CAD build for the part. Positions are in the model's coordinates, mm. Face numbers are marked on the shaded views. A direction names the side the tool comes from. Coordinates: 2 decimals unless noted, no trailing zeros. Loops run counter-clockwise (first coordinate to the right, second up) from the corner with the lowest first, then second, coordinate; pieces in that order, holes last. Notation, with made-up numbers: (13.5, -29) -> (40.5, -29) arc R12 cw to (40.5, -10) -> close; hole circle Ø8 at (44, 76.25). An arc over 180 degrees is marked (long way). Write item = value, one per line. Start each with the question number.
(1) Pull direction Z, two halves, no side cores. Call the marked faces 1, 2, 3 and 4: +Z half, -Z half, draft (parallel to the pull), parting line (faces both ways), or undercut.
(2) Drill centre lines: line 1 (Z direction, x = 5.5, y = 0.5); line 2 (Z direction, x = 10, y = 4.75); line 3 (Z direction, x = 5, y = -1.25). Where is each one in solid material? Low to high. Write a range as from..to.
(3) Band-saw the part on C-C (x = 11.5). Write the cut outline in (y, z).
(4) Flat gauge pins, fed straight in: P1, Ø5, axis at x = 0.5, z = 4, coming from the +Y side; P2, Ø4, axis at y = 2.5, z = 4, coming from the +X side. Where does each tip first touch, or does it go through?
(5) Band-saw the part on A-A (y = 2). Write the cut outline in (x, z).
(6) Tool access for the marked faces 5, 6 and 7: list every direction of +Z, -Z, +X, -X, +Y, -Y with a clear straight run to the whole face (end or side of a thin tool).
(7) Band-saw the part on D-D (x = -1). Write the cut outline in (y, z).
(8) Band-saw the part on B-B (z = 10.5). Write the cut outline in (x, y), and give its area (3 significant figures).
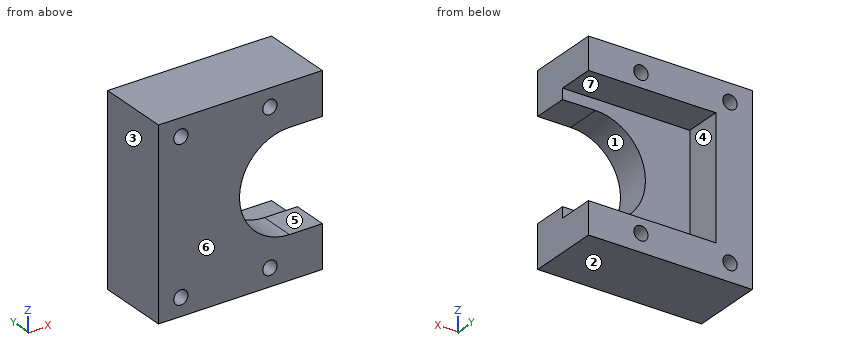
Autodesk Inventor part; units mm, degrees
ref_plane "YZ Plane" through (0, 0, 0) normal (1, 0, 0) x (0, 1, 0)
ref_plane "XZ Plane" through (0, 0, 0) normal (0, 1, 0) x (-1, 0, 0)
ref_plane "XY Plane" through (0, 0, 0) normal (0, 0, 1) x (1, 0, 0)
sketch "スケッチ1" plane through (0, 0, 0) normal (0, 1, 0) x (-1, 0, 0)
  line L0 (10.0552, 13) -> (-14.9448, 13)
  line L1 (-14.9448, 13) -> (-14.9448, -13)
  line L2 (-14.9448, -13) -> (10.0552, -13)
  line L3 (10.0552, -13) -> (10.0552, 13)
  line L4 (10.0552, 0) -> (-14.9448, 0)
  circle A0 centre (6.9152, 10.5) radius 1
  circle A1 centre (6.9152, 10.5) radius 2
  circle A2 centre (-5.5848, 10.5) radius 2
  circle A3 centre (-5.5848, 10.5) radius 1
  circle A4 centre (6.9152, -10.5) radius 2
  circle A5 centre (6.9152, -10.5) radius 1
  circle A6 centre (-5.5848, -10.5) radius 2
  circle A7 centre (-5.5848, -10.5) radius 1
  circle A8 centre (-8.3163, 0) radius 7
  line L5 (-8.3163, 7) -> (-14.9448, 7)
  line L6 (-8.3163, -7) -> (-14.9448, -7)
  line L7 (10.0552, 8.5) -> (-14.9448, 8.5)
  line L8 (4.9152, -13) -> (4.9152, 13)
  line L9 (10.0552, -8.5) -> (-14.9448, -8.5)
  line L10 (-12.9448, 13) -> (-12.9448, -13)
  point P0 (0, 0)
  point P1 (4.9152, 8.5)
  point P2 (4.9152, -8.5)
  point P3 (-5.5848, -8.5)
  point P4 (-5.5848, 8.5)
  point P5 (-12.9448, -8.5)
  point P6 (-12.9448, 8.5)
  point P7 (-12.9448, 7)
  point P8 (-12.9448, -7)
  dimension "d0" = 26
  dimension "d1" = 25
  dimension "d2" = 2
  dimension "d3" = 2.5
  dimension "d4" = 3.14
  dimension "d8" = 12.5
  dimension "d11" = 21
  dimension "d14" = 14
  dimension "d22" = 18.5
  dimension "d23" = 2
extrude "押し出し1" add sketch "スケッチ1" along normal blind 5.2 and the other way blind 5 contours L3 L7 A1 L8 L0 | A2 | L8 L7 L10 L0 | L3 L4 L8 L7 | A1 | A1 L7 L8 | L3 L9 L8 L4 | L3 L2 L8 A4 L9 | A4 | A4 L8 L9 | A6 | L8 L2 L10 L9
extrude "押し出し2" add sketch "スケッチ1" against normal blind 5 contours L3 L7 A1 L8 L0 | L8 L7 L10 L0 | L3 L4 L8 L7 | A1 L7 L8 | L3 L9 L8 L4 | L7 L8 L4 A8 L5 L10 | L3 L2 L8 A4 L9 | L8 L9 L10 L6 A8 L4 | A4 L8 L9 | L8 L2 L10 L9
Findings below:
q1.face_1 = undercut
q1.face_2 = -Z half
q1.face_3 = draft
q1.face_4 = undercut
q2.line_1 = -13..-11.5, -9.5..-8.5, 8.5..9.5, 11.5..13
q2.line_2 = -13..-8.5, 8.5..13
q2.line_3 = -13..-11.31, -9.69..-6.16, 6.16..9.69, 11.31..13
q3.outline = (-5, -13) -> (5.2, -13) -> (5.2, -8.5) -> (0, -8.5) -> (0, -7) -> (-5, -7) -> close; (-5, 7) -> (0, 7) -> (0, 8.5) -> (5.2, 8.5) -> (5.2, 13) -> (-5, 13) -> close
q4.P1 = 0
q4.P2 = -4.92
q5.outline = (-10.06, -13) -> (12.94, -13) -> (12.94, -8.5) -> (-4.92, -8.5) -> (-4.92, 8.5) -> (12.94, 8.5) -> (12.94, 13) -> (-10.06, 13) -> close; hole circle Ø2 at (-6.92, -10.5); hole circle Ø2 at (-6.92, 10.5); hole circle Ø2 at (5.58, -10.5); hole circle Ø2 at (5.58, 10.5)
q6.face_5 = +X, +Y, -Y
q6.face_6 = +Z, -Z, +X, -X, -Y
q6.face_7 = +X, +Y
q7.outline = (-5, -13) -> (5.2, -13) -> (5.2, -8.5) -> (0, -8.5) -> (0, 8.5) -> (5.2, 8.5) -> (5.2, 13) -> (-5, 13) -> close
q8.outline = (-10.06, -5) -> (-7.92, -5) -> (-7.92, 5.2) -> (-10.06, 5.2) -> close; (-5.92, -5) -> (4.58, -5) -> (4.58, 5.2) -> (-5.92, 5.2) -> close; (6.58, -5) -> (12.94, -5) -> (12.94, 5.2) -> (6.58, 5.2) -> close
q8.area = 194 mm²
